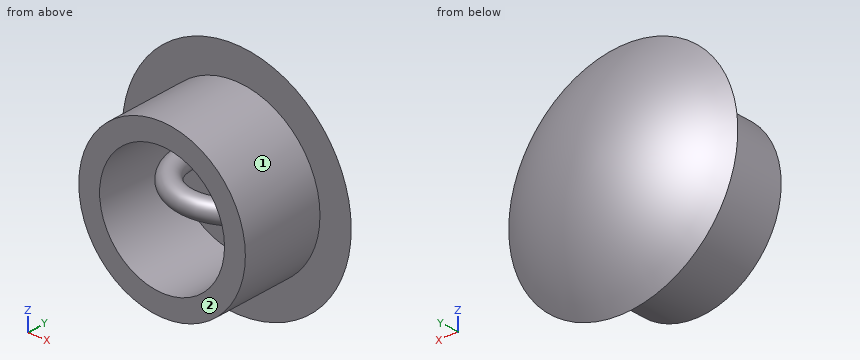
```python
from build123d import *

# Parameters (mm, degrees)
SKETCH1_R           = 6.35
SKETCH1_R_2         = 4.7625
BOSS_EXTRUDE1_DEPTH = 6.35
SKETCH4_R           = 0.79375


with BuildPart() as part:
    # Sketch1 → Boss-Extrude1 (new body)
    with BuildSketch(Plane(origin=(0, 0, 0), x_dir=(1, 0, 0), z_dir=(0, 1, 0))):
        Circle(SKETCH1_R)
        Circle(SKETCH1_R_2, mode=Mode.SUBTRACT)
    extrude(amount=BOSS_EXTRUDE1_DEPTH)

    # Sketch2 → Revolve1 (revolve)
    with BuildSketch(Plane.XY):
        with BuildLine():
            Line((0, 9.525), (0, 6.35))
            Line((0, 6.35), (8.73125, 6.35))
            ThreePointArc((8.73125, 6.35), (4.645302777, 8.706613887), (0, 9.525))
        make_face()
    revolve(axis=Axis((0, 9.525, 0), (0, -1, 0)))

    # Sweep1: sweep along a path in Sketch3
    with BuildLine(Plane.XY) as sweep1_path:
        ThreePointArc((3.862295552, 6.35), (0, 2.487704448), (-3.862295552, 6.35))
    # Sketch4 → Sweep1 (sweep)
    with BuildSketch(Plane.XZ.offset(-6.35)):
        with Locations((3.862295552, 0)):
            Circle(SKETCH4_R)
    sweep(path=sweep1_path.line)


solid = part.part
```
Input: part model. Units: mm. Frame: model coordinates. Face numbers are marked on the shaded views. A direction names the side the tool comes from. Give positions to 0.01 mm unless a question says otherwise; leave off trailing zeros. Loops run counter-clockwise (first coordinate to the right, second up) from the corner with the lowest first, then second, coordinate; pieces in that order, holes last.
1) Section query D-D on y = 5.25. Count the separate pieces of the cut face and the enclosed holes in it, and give its area (3 significant figures).
A:
separate pieces: 3
enclosed holes: 1
area: 59.6 mm2
2) Section query C-C on z = -2.75. Return the cut outline in (x, y).
A:
outline: (-8.29, 6.35) - (-5.72, 6.35) - (-5.72, 0) - (-3.89, 0) - (-3.89, 6.35) - (3.89, 6.35) - (3.89, 0) - (5.72, 0) - (5.72, 6.35) - (8.29, 6.35) arc R13.31 ccw to start
3) Reachability of the marked faces 1 and 2 from +Z, -Z, +X, -X, +Y, -Y: full face, straight path, thin tool, end or side. Return the list, or none.
A:
face 1: -Y
face 2: +Z, -Z, +X, -X, -Y
4) Section query A-A on x = 0. Return the cut outline in (y, z), and give its area (3 significant figures).
A:
outline: (0, -6.35) - (6.35, -6.35) - (6.35, -8.73) arc R13.59 ccw to (6.35, 8.73) - (6.35, 6.35) - (0, 6.35) - (0, 4.76) - (6.35, 4.76) - (6.35, -4.76) - (0, -4.76) - close; circle Ø1.59 at (2.49, 0)
area: 60.1 mm2
5) Line query: L1, parallel to Z at x = 0, y = 3.5; L2, parallel to Z at x = -1.25, y = 2.25. Output: solid intervals per line, ascending.
A:
L1: z = -6.35 to -4.76, 4.76 to 6.35
L2: z = -6.23 to -4.6, -0.67 to 0.67, 4.6 to 6.23
6) Contact query for flat-ended pins moving along their axis: pin 1 (1.5 mm diameter, centred on y = 4.5, z = -5, fed in from +X); pin 2 (2 mm diameter, centred on x = -0.5, y = 1.5, fed in from -Z); pin 3 (4 mm diameter, centred on x = 3, z = -6.5, fed in from +Y). Output: stop coordinate, or through.
A:
pin 1: stops at x = 4.72
pin 2: stops at z = -6.35
pin 3: stops at y = 8.51
